Here's how the part is built. I have some questions about the finished solid (model axes, mm). A direction names the side the tool comes from. Coordinates: 2 decimals unless noted, no trailing zeros. Order: outer loops, then holes, each group sorted by start corner. A loop starts at its lowest first (then second) coordinate and runs counter-clockwise, first axis right, second up. Notation, with made-up numbers: (40, 65) - (94, 65) arc R32 cw to (94, 96) - close; hole circle Ø3 at (51.5, 87). An arc over 180 degrees is marked (long way). Use one line per item in the form item = value. Start each with the question number.
from build123d import *

# Parameters (mm, degrees)
BOSS_EXTRUDE1_DEPTH      = 349.25
BOSS_EXTRUDE1_DEPTH_BACK = 349.25
SKETCH1_W                = 25.4
SKETCH1_H                = 50.8
SKETCH1_W_2              = 19.05
SKETCH1_H_2              = 44.45
CUT_EXTRUDE1_REACH       = 355.624
SKETCH6_R                = 2.4638
CUT_EXTRUDE2_REACH       = 355.624
SKETCH7_R                = 2.4638


with BuildPart() as part:
    # Sketch1 → Boss-Extrude1 (new, two sides: drawn at the far end of the back side and taken through both)
    with BuildSketch(Plane(origin=(0, 0, 0), x_dir=(0, 0, -1), z_dir=(1, 0, 0)).offset(-BOSS_EXTRUDE1_DEPTH_BACK)):
        with Locations((-9.525, 22.225)):
            Rectangle(SKETCH1_W, SKETCH1_H)
        with Locations((-9.525, 22.225)):
            Rectangle(SKETCH1_W_2, SKETCH1_H_2, mode=Mode.SUBTRACT)
    extrude(amount=BOSS_EXTRUDE1_DEPTH + BOSS_EXTRUDE1_DEPTH_BACK)

    # Sketch6 → Cut-Extrude1 (cut, up to next)
    with BuildSketch(Plane(origin=(0, 47.625, 0), x_dir=(1, 0, 0), z_dir=(0, 1, 0)), mode=Mode.PRIVATE) as cut_extrude1_sk1:
        with Locations(Location((330.2, -9.525, 0), (0, 0, 270))):
            Circle(SKETCH6_R)
    cut_extrude1_tool1 = extrude(cut_extrude1_sk1.sketch, amount=-CUT_EXTRUDE1_REACH, mode=Mode.PRIVATE) & part.part
    # Sketch6 → Cut-Extrude1 (cut, up to next)
    with BuildSketch(Plane(origin=(0, 47.625, 0), x_dir=(1, 0, 0), z_dir=(0, 1, 0)), mode=Mode.PRIVATE) as cut_extrude1_sk2:
        with Locations(Location((292.1, -9.525, 0), (0, 0, 270))):
            Circle(SKETCH6_R)
    cut_extrude1_tool2 = extrude(cut_extrude1_sk2.sketch, amount=-CUT_EXTRUDE1_REACH, mode=Mode.PRIVATE) & part.part
    # Sketch6 → Cut-Extrude1 (cut, up to next)
    with BuildSketch(Plane(origin=(0, 47.625, 0), x_dir=(1, 0, 0), z_dir=(0, 1, 0)), mode=Mode.PRIVATE) as cut_extrude1_sk3:
        with Locations(Location((266.7, -9.525, 0), (0, 0, 270))):
            Circle(SKETCH6_R)
    cut_extrude1_tool3 = extrude(cut_extrude1_sk3.sketch, amount=-CUT_EXTRUDE1_REACH, mode=Mode.PRIVATE) & part.part
    # Sketch6 → Cut-Extrude1 (cut, up to next)
    with BuildSketch(Plane(origin=(0, 47.625, 0), x_dir=(1, 0, 0), z_dir=(0, 1, 0)), mode=Mode.PRIVATE) as cut_extrude1_sk4:
        with Locations(Location((241.3, -9.525, 0), (0, 0, 270))):
            Circle(SKETCH6_R)
    cut_extrude1_tool4 = extrude(cut_extrude1_sk4.sketch, amount=-CUT_EXTRUDE1_REACH, mode=Mode.PRIVATE) & part.part
    # Sketch6 → Cut-Extrude1 (cut, up to next)
    with BuildSketch(Plane(origin=(0, 47.625, 0), x_dir=(1, 0, 0), z_dir=(0, 1, 0)), mode=Mode.PRIVATE) as cut_extrude1_sk5:
        with Locations(Location((203.2, -9.525, 0), (0, 0, 270))):
            Circle(SKETCH6_R)
    cut_extrude1_tool5 = extrude(cut_extrude1_sk5.sketch, amount=-CUT_EXTRUDE1_REACH, mode=Mode.PRIVATE) & part.part
    # Sketch6 → Cut-Extrude1 (cut, up to next)
    with BuildSketch(Plane(origin=(0, 47.625, 0), x_dir=(1, 0, 0), z_dir=(0, 1, 0)), mode=Mode.PRIVATE) as cut_extrude1_sk6:
        with Locations(Location((76.2, -9.525, 0), (0, 0, 270))):
            Circle(SKETCH6_R)
    cut_extrude1_tool6 = extrude(cut_extrude1_sk6.sketch, amount=-CUT_EXTRUDE1_REACH, mode=Mode.PRIVATE) & part.part
    # Sketch6 → Cut-Extrude1 (cut, up to next)
    with BuildSketch(Plane(origin=(0, 47.625, 0), x_dir=(1, 0, 0), z_dir=(0, 1, 0)), mode=Mode.PRIVATE) as cut_extrude1_sk7:
        with Locations(Location((38.1, -9.525, 0), (0, 0, 270))):
            Circle(SKETCH6_R)
    cut_extrude1_tool7 = extrude(cut_extrude1_sk7.sketch, amount=-CUT_EXTRUDE1_REACH, mode=Mode.PRIVATE) & part.part
    # Sketch6 → Cut-Extrude1 (cut, up to next)
    with BuildSketch(Plane(origin=(0, 47.625, 0), x_dir=(1, 0, 0), z_dir=(0, 1, 0)), mode=Mode.PRIVATE) as cut_extrude1_sk8:
        with Locations(Location((12.7, -9.525, 0), (0, 0, 270))):
            Circle(SKETCH6_R)
    cut_extrude1_tool8 = extrude(cut_extrude1_sk8.sketch, amount=-CUT_EXTRUDE1_REACH, mode=Mode.PRIVATE) & part.part
    # Sketch6 → Cut-Extrude1 (cut, up to next)
    with BuildSketch(Plane(origin=(0, 47.625, 0), x_dir=(1, 0, 0), z_dir=(0, 1, 0)), mode=Mode.PRIVATE) as cut_extrude1_sk9:
        with Locations(Location((-12.7, -9.525, 0), (0, 0, 270))):
            Circle(SKETCH6_R)
    cut_extrude1_tool9 = extrude(cut_extrude1_sk9.sketch, amount=-CUT_EXTRUDE1_REACH, mode=Mode.PRIVATE) & part.part
    # Sketch6 → Cut-Extrude1 (cut, up to next)
    with BuildSketch(Plane(origin=(0, 47.625, 0), x_dir=(1, 0, 0), z_dir=(0, 1, 0)), mode=Mode.PRIVATE) as cut_extrude1_sk10:
        with Locations(Location((-38.1, -9.525, 0), (0, 0, 270))):
            Circle(SKETCH6_R)
    cut_extrude1_tool10 = extrude(cut_extrude1_sk10.sketch, amount=-CUT_EXTRUDE1_REACH, mode=Mode.PRIVATE) & part.part
    # Sketch6 → Cut-Extrude1 (cut, up to next)
    with BuildSketch(Plane(origin=(0, 47.625, 0), x_dir=(1, 0, 0), z_dir=(0, 1, 0)), mode=Mode.PRIVATE) as cut_extrude1_sk11:
        with Locations(Location((-76.2, -9.525, 0), (0, 0, 270))):
            Circle(SKETCH6_R)
    cut_extrude1_tool11 = extrude(cut_extrude1_sk11.sketch, amount=-CUT_EXTRUDE1_REACH, mode=Mode.PRIVATE) & part.part
    # Sketch6 → Cut-Extrude1 (cut, up to next)
    with BuildSketch(Plane(origin=(0, 47.625, 0), x_dir=(1, 0, 0), z_dir=(0, 1, 0)), mode=Mode.PRIVATE) as cut_extrude1_sk12:
        with Locations(Location((-203.2, -9.525, 0), (0, 0, 270))):
            Circle(SKETCH6_R)
    cut_extrude1_tool12 = extrude(cut_extrude1_sk12.sketch, amount=-CUT_EXTRUDE1_REACH, mode=Mode.PRIVATE) & part.part
    # Sketch6 → Cut-Extrude1 (cut, up to next)
    with BuildSketch(Plane(origin=(0, 47.625, 0), x_dir=(1, 0, 0), z_dir=(0, 1, 0)), mode=Mode.PRIVATE) as cut_extrude1_sk13:
        with Locations(Location((-241.3, -9.525, 0), (0, 0, 270))):
            Circle(SKETCH6_R)
    cut_extrude1_tool13 = extrude(cut_extrude1_sk13.sketch, amount=-CUT_EXTRUDE1_REACH, mode=Mode.PRIVATE) & part.part
    # Sketch6 → Cut-Extrude1 (cut, up to next)
    with BuildSketch(Plane(origin=(0, 47.625, 0), x_dir=(1, 0, 0), z_dir=(0, 1, 0)), mode=Mode.PRIVATE) as cut_extrude1_sk14:
        with Locations(Location((-330.2, -9.525, 0), (0, 0, 270))):
            Circle(SKETCH6_R)
    cut_extrude1_tool14 = extrude(cut_extrude1_sk14.sketch, amount=-CUT_EXTRUDE1_REACH, mode=Mode.PRIVATE) & part.part
    # Sketch6 → Cut-Extrude1 (cut, up to next)
    with BuildSketch(Plane(origin=(0, 47.625, 0), x_dir=(1, 0, 0), z_dir=(0, 1, 0)), mode=Mode.PRIVATE) as cut_extrude1_sk15:
        with Locations(Location((-292.1, -9.525, 0), (0, 0, 270))):
            Circle(SKETCH6_R)
    cut_extrude1_tool15 = extrude(cut_extrude1_sk15.sketch, amount=-CUT_EXTRUDE1_REACH, mode=Mode.PRIVATE) & part.part
    # Sketch6 → Cut-Extrude1 (cut, up to next)
    with BuildSketch(Plane(origin=(0, 47.625, 0), x_dir=(1, 0, 0), z_dir=(0, 1, 0)), mode=Mode.PRIVATE) as cut_extrude1_sk16:
        with Locations(Location((-266.7, -9.525, 0), (0, 0, 270))):
            Circle(SKETCH6_R)
    cut_extrude1_tool16 = extrude(cut_extrude1_sk16.sketch, amount=-CUT_EXTRUDE1_REACH, mode=Mode.PRIVATE) & part.part
    add(cut_extrude1_tool1.solids().sort_by_distance((330.2, 47.625, 9.525))[0], mode=Mode.SUBTRACT)
    add(cut_extrude1_tool2.solids().sort_by_distance((292.1, 47.625, 9.525))[0], mode=Mode.SUBTRACT)
    add(cut_extrude1_tool3.solids().sort_by_distance((266.7, 47.625, 9.525))[0], mode=Mode.SUBTRACT)
    add(cut_extrude1_tool4.solids().sort_by_distance((241.3, 47.625, 9.525))[0], mode=Mode.SUBTRACT)
    add(cut_extrude1_tool5.solids().sort_by_distance((203.2, 47.625, 9.525))[0], mode=Mode.SUBTRACT)
    add(cut_extrude1_tool6.solids().sort_by_distance((76.2, 47.625, 9.525))[0], mode=Mode.SUBTRACT)
    add(cut_extrude1_tool7.solids().sort_by_distance((38.1, 47.625, 9.525))[0], mode=Mode.SUBTRACT)
    add(cut_extrude1_tool8.solids().sort_by_distance((12.7, 47.625, 9.525))[0], mode=Mode.SUBTRACT)
    add(cut_extrude1_tool9.solids().sort_by_distance((-12.7, 47.625, 9.525))[0], mode=Mode.SUBTRACT)
    add(cut_extrude1_tool10.solids().sort_by_distance((-38.1, 47.625, 9.525))[0], mode=Mode.SUBTRACT)
    add(cut_extrude1_tool11.solids().sort_by_distance((-76.2, 47.625, 9.525))[0], mode=Mode.SUBTRACT)
    add(cut_extrude1_tool12.solids().sort_by_distance((-203.2, 47.625, 9.525))[0], mode=Mode.SUBTRACT)
    add(cut_extrude1_tool13.solids().sort_by_distance((-241.3, 47.625, 9.525))[0], mode=Mode.SUBTRACT)
    add(cut_extrude1_tool14.solids().sort_by_distance((-330.2, 47.625, 9.525))[0], mode=Mode.SUBTRACT)
    add(cut_extrude1_tool15.solids().sort_by_distance((-292.1, 47.625, 9.525))[0], mode=Mode.SUBTRACT)
    add(cut_extrude1_tool16.solids().sort_by_distance((-266.7, 47.625, 9.525))[0], mode=Mode.SUBTRACT)

    # Sketch7 → Cut-Extrude2 (cut, up to next)
    with BuildSketch(Plane(origin=(0, -3.175, 0), x_dir=(-1, 0, 0), z_dir=(0, -1, 0)), mode=Mode.PRIVATE) as cut_extrude2_sk1:
        with Locations(Location((-266.7, -9.525, 0), (0, 0, 270))):
            Circle(SKETCH7_R)
    cut_extrude2_tool1 = extrude(cut_extrude2_sk1.sketch, amount=-CUT_EXTRUDE2_REACH, mode=Mode.PRIVATE) & part.part
    # Sketch7 → Cut-Extrude2 (cut, up to next)
    with BuildSketch(Plane(origin=(0, -3.175, 0), x_dir=(-1, 0, 0), z_dir=(0, -1, 0)), mode=Mode.PRIVATE) as cut_extrude2_sk2:
        with Locations(Location((-190.5, -9.525, 0), (0, 0, 90))):
            Circle(SKETCH7_R)
    cut_extrude2_tool2 = extrude(cut_extrude2_sk2.sketch, amount=-CUT_EXTRUDE2_REACH, mode=Mode.PRIVATE) & part.part
    # Sketch7 → Cut-Extrude2 (cut, up to next)
    with BuildSketch(Plane(origin=(0, -3.175, 0), x_dir=(-1, 0, 0), z_dir=(0, -1, 0)), mode=Mode.PRIVATE) as cut_extrude2_sk3:
        with Locations(Location((-114.3, -9.525, 0), (0, 0, 90))):
            Circle(SKETCH7_R)
    cut_extrude2_tool3 = extrude(cut_extrude2_sk3.sketch, amount=-CUT_EXTRUDE2_REACH, mode=Mode.PRIVATE) & part.part
    # Sketch7 → Cut-Extrude2 (cut, up to next)
    with BuildSketch(Plane(origin=(0, -3.175, 0), x_dir=(-1, 0, 0), z_dir=(0, -1, 0)), mode=Mode.PRIVATE) as cut_extrude2_sk4:
        with Locations(Location((-38.1, -9.525, 0), (0, 0, 270))):
            Circle(SKETCH7_R)
    cut_extrude2_tool4 = extrude(cut_extrude2_sk4.sketch, amount=-CUT_EXTRUDE2_REACH, mode=Mode.PRIVATE) & part.part
    # Sketch7 → Cut-Extrude2 (cut, up to next)
    with BuildSketch(Plane(origin=(0, -3.175, 0), x_dir=(-1, 0, 0), z_dir=(0, -1, 0)), mode=Mode.PRIVATE) as cut_extrude2_sk5:
        with Locations(Location((38.1, -9.525, 0), (0, 0, 270))):
            Circle(SKETCH7_R)
    cut_extrude2_tool5 = extrude(cut_extrude2_sk5.sketch, amount=-CUT_EXTRUDE2_REACH, mode=Mode.PRIVATE) & part.part
    # Sketch7 → Cut-Extrude2 (cut, up to next)
    with BuildSketch(Plane(origin=(0, -3.175, 0), x_dir=(-1, 0, 0), z_dir=(0, -1, 0)), mode=Mode.PRIVATE) as cut_extrude2_sk6:
        with Locations(Location((114.3, -9.525, 0), (0, 0, 90))):
            Circle(SKETCH7_R)
    cut_extrude2_tool6 = extrude(cut_extrude2_sk6.sketch, amount=-CUT_EXTRUDE2_REACH, mode=Mode.PRIVATE) & part.part
    # Sketch7 → Cut-Extrude2 (cut, up to next)
    with BuildSketch(Plane(origin=(0, -3.175, 0), x_dir=(-1, 0, 0), z_dir=(0, -1, 0)), mode=Mode.PRIVATE) as cut_extrude2_sk7:
        with Locations(Location((190.5, -9.525, 0), (0, 0, 90))):
            Circle(SKETCH7_R)
    cut_extrude2_tool7 = extrude(cut_extrude2_sk7.sketch, amount=-CUT_EXTRUDE2_REACH, mode=Mode.PRIVATE) & part.part
    # Sketch7 → Cut-Extrude2 (cut, up to next)
    with BuildSketch(Plane(origin=(0, -3.175, 0), x_dir=(-1, 0, 0), z_dir=(0, -1, 0)), mode=Mode.PRIVATE) as cut_extrude2_sk8:
        with Locations(Location((266.7, -9.525, 0), (0, 0, 270))):
            Circle(SKETCH7_R)
    cut_extrude2_tool8 = extrude(cut_extrude2_sk8.sketch, amount=-CUT_EXTRUDE2_REACH, mode=Mode.PRIVATE) & part.part
    add(cut_extrude2_tool1.solids().sort_by_distance((266.7, -3.175, 9.525))[0], mode=Mode.SUBTRACT)
    add(cut_extrude2_tool2.solids().sort_by_distance((190.5, -3.175, 9.525))[0], mode=Mode.SUBTRACT)
    add(cut_extrude2_tool3.solids().sort_by_distance((114.3, -3.175, 9.525))[0], mode=Mode.SUBTRACT)
    add(cut_extrude2_tool4.solids().sort_by_distance((38.1, -3.175, 9.525))[0], mode=Mode.SUBTRACT)
    add(cut_extrude2_tool5.solids().sort_by_distance((-38.1, -3.175, 9.525))[0], mode=Mode.SUBTRACT)
    add(cut_extrude2_tool6.solids().sort_by_distance((-114.3, -3.175, 9.525))[0], mode=Mode.SUBTRACT)
    add(cut_extrude2_tool7.solids().sort_by_distance((-190.5, -3.175, 9.525))[0], mode=Mode.SUBTRACT)
    add(cut_extrude2_tool8.solids().sort_by_distance((-266.7, -3.175, 9.525))[0], mode=Mode.SUBTRACT)


solid = part.part
1) Suppose I cut it at A-A, the plane y = 9.5. List the corners of the cut face in (x, z) for me (3 decimals), then the cut area to 3 significant figures.
2) If we mould it in two halves opening along Z, with no side actions, what happens to faces 1 (the flat face through (-5, 22, 0)), 2 (the flat face through (-5, -3.175, 10)), 3 (the flat face through (-5, 22, -3.175)), 4 (the flat face through (-5, 0, 10))? For each: pulls with the +Z half, pulls with the -Z half, needs draft (parallel to the pull), parting line crosses it, or undercut.
3) Suppose I cut it at B-B, the plane x = -181. List the corners of the cut face in (y, z) for me (3 decimals), then the cut area to 3 significant figures.
4) For pin 1 (8 mm diameter, centred on x = 266.7, z = 9.525, fed in from -Y) (3 decimals); pin 2 (4 mm diameter, centred on x = -114.3, z = 9.525, fed in from -Y), each with a flat end and sliding along its axis, tell me the tip position at first contact or that it passes through.
5) Which directions (+Z, -Z, +X, -X, +Y, -Y) give clear straight access to the entire face, cutting with the end or side of a thin tool? Please do faces 5 (the flat face through (349.25, 20, 20)), 6 (the flat face through (-5, 22, 19.05)).
6) I need wall thicknesses on probe 1 along Y at (x, z) = (307.5, 18) (3 decimals); probe 2 along Z at (x, y) = (-271, 5.5) (3 decimals); probe 3 along Z at (x, y) = (-203.2, 46.1) (3 decimals). Which ranges of each line are inside material? Lowest first, please. Write a range as [from, to].
From the geometry:
q1.outline = (-349.25, -3.175) - (349.25, -3.175) - (349.25, 0) - (-349.25, 0) - close; (-349.25, 19.05) - (349.25, 19.05) - (349.25, 22.225) - (-349.25, 22.225) - close
q1.area = 4,440 mm2
q2.face_1 = undercut
q2.face_2 = needs draft
q2.face_3 = pulls with the -Z half
q2.face_4 = undercut
q3.outline = (-3.175, -3.175) - (47.625, -3.175) - (47.625, 22.225) - (-3.175, 22.225) - close; hole (0, 0) - (44.45, 0) - (44.45, 19.05) - (0, 19.05) - close
q3.area = 444 mm2
q4.pin_1 = -3.175
q4.pin_2 = 44.45
q5.face_5 = +Z, -Z, +X, +Y, -Y
q5.face_6 = +X, -X
q6.probe_1 = [-3.175, 0], [44.45, 47.625]
q6.probe_2 = [-3.175, 0], [19.05, 22.225]
q6.probe_3 = [-3.175, 7.061], [11.989, 22.225]
